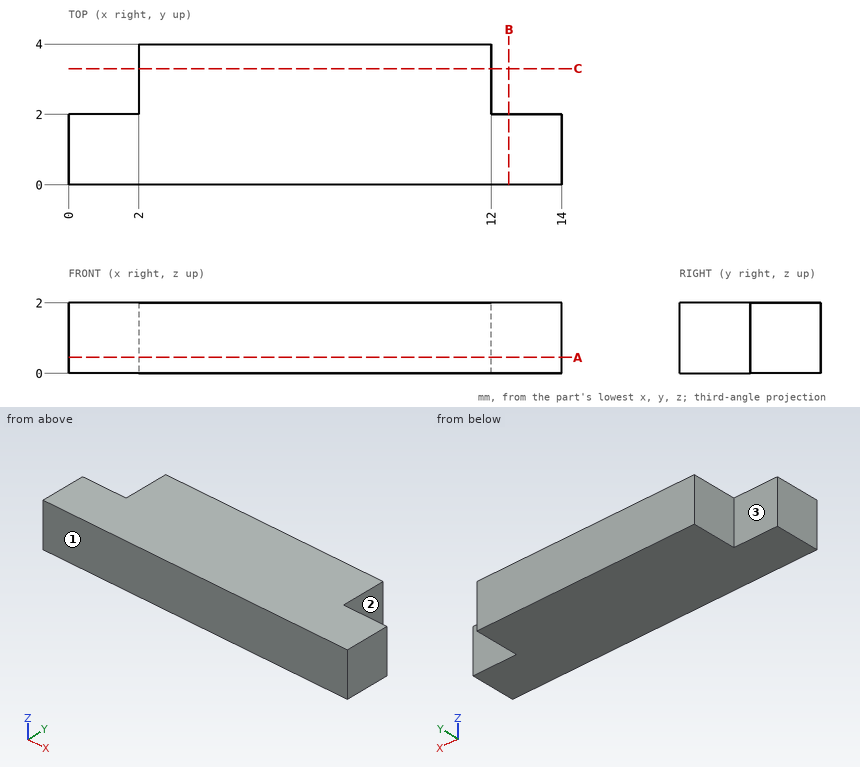
Geometry check sheet. Reference: drawing and pictorial views, mm from the part's lowest x, y, z. A direction names the side the tool comes from. Coordinates: 2 decimals unless noted, no trailing zeros. Loops run counter-clockwise (first coordinate to the right, second up) from the corner with the lowest first, then second, coordinate; pieces in that order, holes last.
1) Material ranges on probe 1 along Y at (x, z) = (13.25, 0.95); probe 2 along X at (y, z) = (3.7, 0.6), recorded low to high.
2) Sectioned sample at B-B (x = 12.5). Record the boundary of the cut face in (y, z).
3) Gauge pin test, flat ends, axial feed: pin 1 (1 mm diameter, centred on y = 3.5, z = 1.5, fed in from -X); pin 2 (1 mm diameter, centred on y = 3.5, z = 0.5, fed in from +X); pin 3 (1 mm diameter, centred on x = 13.5, z = 1, fed in from +Y). Record the tip position at first contact, or that the pin passes through.
4) Sectioned sample at A-A (z = 0.45). Record the boundary of the cut face in (x, y), and give its area (3 significant figures).
5) Access from +Z, -Z, +X, -X, +Y, -Y to the whole of each face (thin tool, end or side, straight path). Record for the marked faces 1, 2 and 3.
6) Sectioned sample at C-C (y = 3.3). Record the boundary of the cut face in (x, z).
Check sheet entries:
1. probe 1: y = 0 to 2
1. probe 2: x = 2 to 12
2. outline: (0, 0) - (2, 0) - (2, 2) - (0, 2) - close
3. pin 1: stops at x = 2
3. pin 2: stops at x = 12
3. pin 3: stops at y = 2
4. outline: (0, 0) - (14, 0) - (14, 2) - (12, 2) - (12, 4) - (2, 4) - (2, 2) - (0, 2) - close
4. area: 48.0 mm2
5. face 1: +Z, -Z, +X, -X, -Y
5. face 2: +Z, -Z, +X, +Y
5. face 3: +Z, -Z, -X, +Y
6. outline: (2, 0) - (12, 0) - (12, 2) - (2, 2) - close
